Geometry check sheet. Reference: drawing and pictorial views, mm from the part's lowest x, y, z. A direction names the side the tool comes from. Round coordinates to 2 decimals unless told otherwise and drop trailing zeros. Loops run counter-clockwise (first coordinate to the right, second up) from the corner with the lowest first, then second, coordinate; pieces in that order, holes last. Notation, with made-up numbers: (71, 81.5) - (106, 81.5) arc R25 ccw to (106, 117.5) - close; hole circle Ø1 at (-25.5, 46). An arc over 180 degrees is marked (long way). Put each result on its own line as item: value. Start each with the question number.
Item 1: Section check C-C, the plane z = 63.5. Record the cut outline in (x, y) (3 decimals).
Item 2: Section check D-D, the plane x = 137.5. Record the cut outline in (y, z), and give its area (3 significant figures).
Item 3: Tool access check on the marked faces 1 and 2. Record the directions out of +Z, -Z, +X, -X, +Y, -Y that give a thin tool (end or side, any length) a straight path to the whole face; none if there is none.
Item 4: Material ranges on line 1 along Y through (x, z) = (38.1, 10) (3 decimals); line 2 along Z through (x, y) = (38, 104); line 3 along X through (y, z) = (76, 9), recorded low to high.
Item 5: Gauge pin test, flat ends, axial feed: pin 1 Ø8 at (x, z) = (78, 177.5) entering from -Y; pin 2 Ø25 at (x, y) = (114.3, 25.4) entering from +Z. Record the tip position at first contact, or that the pin passes through.
Item 6: Section check B-B, the plane y = 76.2. Record the cut outline in (x, z) (3 decimals), and give its area (3 significant figures).
Item 7: Section check A-A, the plane x = 114.3. Record the cut outline in (y, z) (3 decimals), and give its area (3 significant figures).
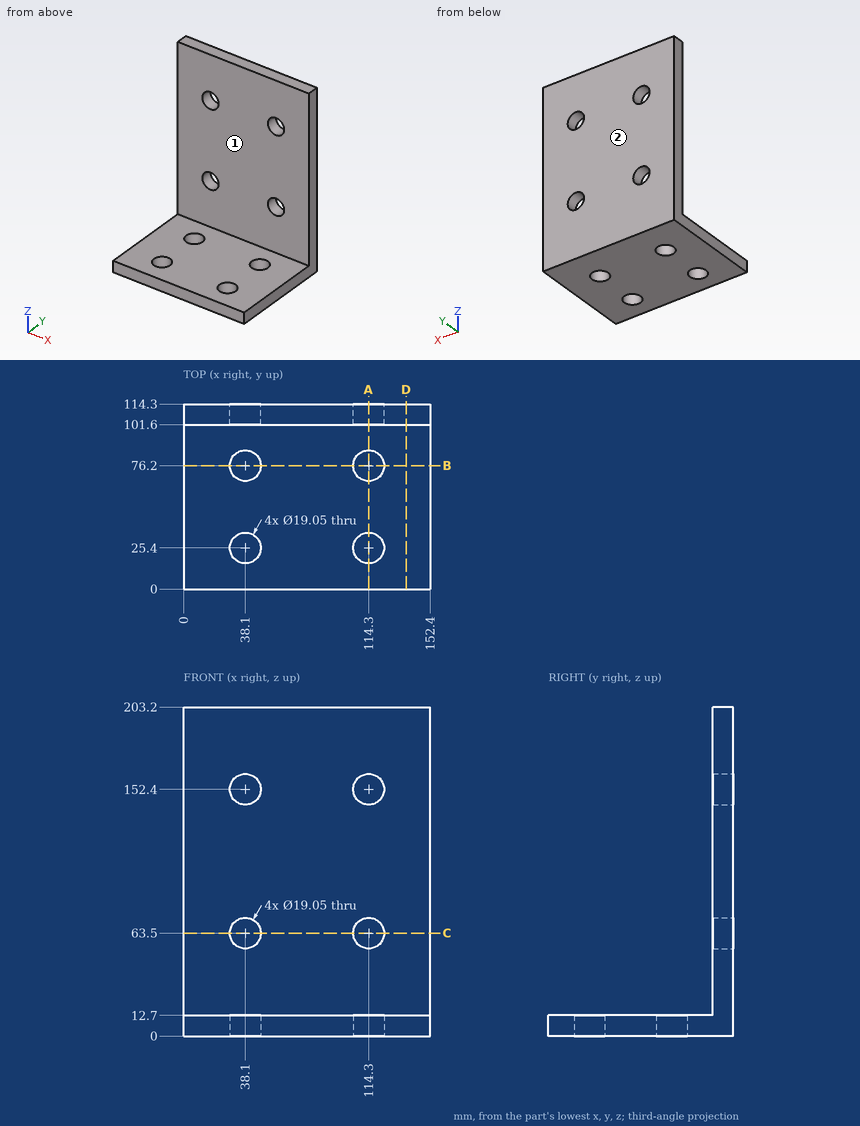
Check result:
1. outline: (0, 101.6) - (28.575, 101.6) - (28.575, 114.3) - (0, 114.3) - close; (47.625, 101.6) - (104.775, 101.6) - (104.775, 114.3) - (47.625, 114.3) - close; (123.825, 101.6) - (152.4, 101.6) - (152.4, 114.3) - (123.825, 114.3) - close
2. outline: (0, 0) - (114.3, 0) - (114.3, 203.2) - (101.6, 203.2) - (101.6, 12.7) - (0, 12.7) - close
2. area: 3,870 mm²
3. face 1: +Z, +X, -X, -Y
3. face 2: +Z, -Z, +X, -X, +Y
4. line 1: 0 to 15.875, 34.925 to 66.675, 85.725 to 114.3
4. line 2: 0 to 53.98, 73.02 to 142.88, 161.92 to 203.2
4. line 3: 0 to 28.58, 47.62 to 104.78, 123.82 to 152.4
5. pin 1: y = 101.6
5. pin 2: z = 12.7
6. outline: (0, 0) - (28.575, 0) - (28.575, 12.7) - (0, 12.7) - close; (47.625, 0) - (104.775, 0) - (104.775, 12.7) - (47.625, 12.7) - close; (123.825, 0) - (152.4, 0) - (152.4, 12.7) - (123.825, 12.7) - close
6. area: 1,450 mm²
7. outline: (0, 0) - (15.875, 0) - (15.875, 12.7) - (0, 12.7) - close; (34.925, 0) - (66.675, 0) - (66.675, 12.7) - (34.925, 12.7) - close; (85.725, 0) - (114.3, 0) - (114.3, 53.975) - (101.6, 53.975) - (101.6, 12.7) - (85.725, 12.7) - close; (101.6, 73.025) - (114.3, 73.025) - (114.3, 142.875) - (101.6, 142.875) - close; (101.6, 161.925) - (114.3, 161.925) - (114.3, 203.2) - (101.6, 203.2) - close
7. area: 2,900 mm²
